Work out the finished part from the listing and answer in its coordinate system (mm). Face numbers are marked on the shaded views. A direction names the side the tool comes from. Coordinates: 2 decimals unless noted, no trailing zeros. Order: outer loops, then holes, each group sorted by start corner. A loop starts at its lowest first (then second) coordinate and runs counter-clockwise, first axis right, second up. Notation, with made-up numbers: M 8.5,53.5 L 30.5,53.5 A15 ccw 30.5,57.5 Z; hole C -14.75,-2 d7. An arc over 180 degrees is marked long. Answer in a Markdown table with one row per item. Add a question column.
Item 1: The part is cut by section B-B (x = 66.5). Write down the section's boundary in (y, z), then the cut area to 3 significant figures.
Item 2: The part is cut by section C-C (x = -55). Write down the section's boundary in (y, z), then the cut area to 3 significant figures.
Item 3: Which of the six approach directions +Z, -Z, +X, -X, +Y, -Y give full straight-line access (tool end or side, diameter ignored) to the marked faces 1 and 2?
Item 4: The mould has two halves that part along Z. Classify the marked faces 3, 4 and 5: released by +Z, released by -Z, zero draft, split by the parting line, or undercut.
Item 5: The part is cut by section A-A (z = 0). Write down the section's boundary in (x, y), then the cut area to 4 significant figures.
Item 6: Consider line 1 (Z direction, x = -35, y = 1); line 2 (X direction, y = 0.5, z = 0.5); line 3 (Z direction, x = 53, y = 0.75). Determine where each line is inside the solid, lowest interval first. Write a range as from..to.
Item 7: The part is cut by section D-D (y = -0.25). Write down the section's boundary in (x, z), then the cut area to 3 significant figures.
Autodesk Inventor part; units mm, degrees
ref_plane "YZ Plane" through (0, 0, 0) normal (1, 0, 0) x (0, 1, 0)
ref_plane "XZ Plane" through (0, 0, 0) normal (0, 1, 0) x (-1, 0, 0)
ref_plane "XY Plane" through (0, 0, 0) normal (0, 0, 1) x (1, 0, 0)
sketch "Sketch1" plane through (0, 0, 0) normal (0, 1, 0) x (-1, 0, 0)
  line L0 (-75, 30) -> (75, 30)
  line L1 (75, 30) -> (75, -30)
  line L2 (75, -30) -> (-75, -30)
  line L3 (-75, -30) -> (-75, 30)
  line L4 (-75, 30) -> (75, -30) construction
  line L5 (75, 30) -> (-75, -30) construction
  line L6 (-80, 0) -> (-40, 0) construction
  line L7 (-80, -8.5) -> (-40, -8.5)
  line L8 (-40, 8.5) -> (-80, 8.5)
  arc A0 (-80, 8.5) -> (-80, -8.5) centre (-80, 0) ccw
  arc A1 (-40, -8.5) -> (-40, 8.5) centre (-40, 0) ccw
  circle A2 centre (55, 15) radius 3.5
  circle A3 centre (55, -15) radius 3.5
  circle A4 centre (35, 15) radius 3.5
  circle A5 centre (35, -15) radius 3.5
  point P0 (0, 0)
  point P1 (-60, 0)
  dimension "d0" = 60
  dimension "d1" = 150
  dimension "d2" = 60
  dimension "d3" = 40
  dimension "d4" = 17
  dimension "d5" = 7
  dimension "d6" = 15
  dimension "d7" = 30
  dimension "d8" = 20
  dimension "d9" = 20
extrude "Plate1" add sketch "Sketch1" along normal mid plane 10 contours L0 L1 L2 L3 L7 A1 L8 | L8 A1 L7 L3
extrude "Cut1" cut sketch "Sketch1" against normal mid plane 10 contours L8 A1 L7 L3 | L3 L7 A0 L8
sketch "Sketch2" plane through (0, -5, 0) normal (0, -1, 0) x (1, 0, 0)
  line L0 (-3, 12) -> (3, 12)
  line L1 (3, 12) -> (3, -12)
  line L2 (3, -12) -> (-3, -12)
  line L3 (-3, -12) -> (-3, 12)
  line L4 (75, 30) -> (-75, 30)
  point P0 (0, 0)
  point P1 (0, 12)
  dimension "d13" = 24
  dimension "d14" = 18
  dimension "d15" = 6
extrude "Cut2" cut sketch "Sketch2" against normal blind 10
fillet "Corner Round1" radius 6 4 edges at (75, 0, 30) (75, 0, 8.5) (75, 0, -8.5) (75, 0, -30)
equation "\"d11\" = Thickness"
equation "\"d16\" = Thickness"
equation "\"d10\" = Thickness"
equation "\"BendReliefDepth\" = 0.5 * Thickness"
properties part number "HCMUTE-CDT23-BAT_TRUC_CANG_TAI" material "Stainless Steel"
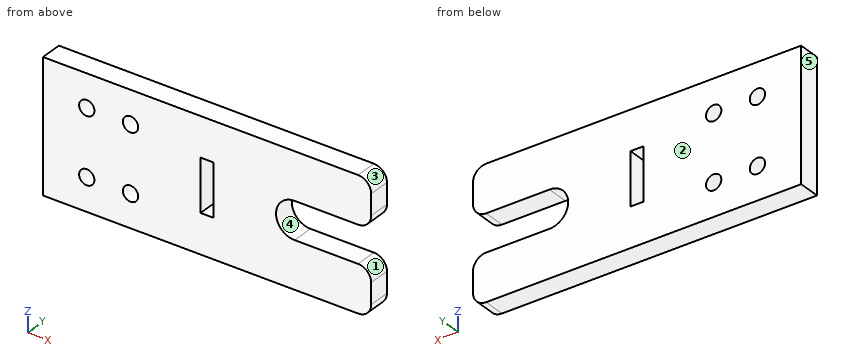
Reply:
| question | item | result |
|---|---|---|
| 1 | outline | M -5,-30 L 5,-30 L 5,-8.5 L -5,-8.5 Z; M -5,8.5 L 5,8.5 L 5,30 L -5,30 Z |
| 1 | area | 430 mm2 |
| 2 | outline | M -5,-30 L 5,-30 L 5,-18.5 L -5,-18.5 Z; M -5,-11.5 L 5,-11.5 L 5,11.5 L -5,11.5 Z; M -5,18.5 L 5,18.5 L 5,30 L -5,30 Z |
| 2 | area | 460 mm2 |
| 3 | face 1 | +X, +Y, -Y |
| 3 | face 2 | +Z, -Z, +X, -X, +Y |
| 4 | face 3 | released by +Z |
| 4 | face 4 | undercut |
| 4 | face 5 | zero draft |
| 5 | outline | M -75,-5 L -3,-5 L -3,5 L -75,5 Z; M 3,-5 L 31.5,-5 L 31.5,5 L 3,5 Z |
| 5 | area | 1,005 mm2 |
| 6 | line 1 | z = -30..-18.5, -11.5..11.5, 18.5..30 |
| 6 | line 2 | x = -75..-3, 3..31.51 |
| 6 | line 3 | z = -30..-8.5, 8.5..30 |
| 7 | outline | M -75,-30 L 69,-30 A6 ccw 75,-24 L 75,-14.5 A6 ccw 69,-8.5 L 40,-8.5 A8.5 cw 40,8.5 L 69,8.5 A6 ccw 75,14.5 L 75,24 A6 ccw 69,30 L -75,30 Z; hole C -55,-15 d7; hole C -55,15 d7; hole C -35,-15 d7; hole C -35,15 d7; hole M -3,-12 L 3,-12 L 3,12 L -3,12 Z |
| 7 | area | 7,960 mm2 |
